Could you check a few things on this model? Use its own coordinates, in mm. A direction names the side the tool comes from. Coordinates: 2 decimals unless noted, no trailing zeros. Write each loop counter-clockwise with the first axis right and the second up, starting at its lowest first coordinate (ties: lowest second). Pieces come first, ordered by that corner, then holes. Notation, with made-up numbers: M 43,-38 L 65,-38 A11 cw 65,-20 Z; hole C -21.75,-36 d4. An arc over 180 degrees is marked long. Write item = value, one per line.
```python
from build123d import *

# Parameters (mm, degrees)
SKETCH4_W               = 40
SKETCH4_H               = 80
BOSS_EXTRUDE4_DEPTH     = 5
SKETCH5_W               = 10
SKETCH5_H               = 5
BOSS_EXTRUDE6_DEPTH     = 50
SKETCH7_W               = 10
SKETCH7_H               = 25
SKETCH7_H_2             = 5
BOSS_EXTRUDE7_DEPTH     = 20
SKETCH8_W               = 40
SKETCH8_H               = 5
BOSS_EXTRUDE8_DEPTH     = 20
SKETCH9_W               = 100
SKETCH9_H               = 5
BOSS_EXTRUDE9_DEPTH     = 10
SKETCH10_W              = 5
SKETCH10_H              = 50
BOSS_EXTRUDE10_DEPTH    = 40
BOSS_EXTRUDE11_DEPTH    = 10
SKETCH12_R              = 15
SKETCH12_R_2            = 1.8
CUT_EXTRUDE1_DEPTH      = 5
CUT_EXTRUDE2_DEPTH      = 92.241437954
CUT_EXTRUDE2_DEPTH_BACK = 92.241437954
SKETCH13_R              = 2.25
SKETCH14_R              = 4
SKETCH14_R_2            = 2.25
CUT_EXTRUDE4_DEPTH      = 2
CUT_EXTRUDE5_START      = -2
SKETCH15_R              = 4
SKETCH15_R_2            = 2.25
CUT_EXTRUDE5_DEPTH      = 2
SKETCH17_R              = 5
CUT_EXTRUDE6_DEPTH      = 25
SKETCH19_W              = 50
SKETCH19_H              = 60
SKETCH19_R              = 1.8
SKETCH19_R_2            = 15
SKETCH19_R_3            = 4
BOSS_EXTRUDE13_DEPTH    = 5
SKETCH20_R              = 4
SKETCH20_R_2            = 2.25
BOSS_EXTRUDE14_DEPTH    = 5
SKETCH21_W              = 20
SKETCH21_H              = 20
BOSS_EXTRUDE15_DEPTH    = 5
BOSS_EXTRUDE16_START    = -10
SKETCH22_R              = 4
BOSS_EXTRUDE16_DEPTH    = 10
SKETCH23_R              = 4
BOSS_EXTRUDE17_DEPTH    = 5
CUT_EXTRUDE7_DEPTH      = 106.59356041
CUT_EXTRUDE7_DEPTH_BACK = 106.59356041
SKETCH24_R              = 2.6
SKETCH25_W              = 55
SKETCH25_H              = 100
BOSS_EXTRUDE18_DEPTH    = 5
SKETCH26_W              = 55
SKETCH26_H              = 10
BOSS_EXTRUDE19_DEPTH    = 20


with BuildPart() as part:
    # Sketch4 → Boss-Extrude4 (new body)
    with BuildSketch(Plane(origin=(0, 0, 0), x_dir=(1, 0, 0), z_dir=(0, 1, 0))):
        with Locations((20, 40)):
            Rectangle(SKETCH4_W, SKETCH4_H)
    extrude(amount=BOSS_EXTRUDE4_DEPTH)

    # Sketch5 → Boss-Extrude6 (add)
    with BuildSketch(Plane(origin=(0, 5, 0), x_dir=(1, 0, 0), z_dir=(0, 1, 0))):
        with Locations((35, 52.5)):
            Rectangle(SKETCH5_W, SKETCH5_H)
        with Locations((35, 27.5)):
            Rectangle(SKETCH5_W, SKETCH5_H)
    extrude(amount=BOSS_EXTRUDE6_DEPTH)

    # Sketch7 → Boss-Extrude7 (add)
    with BuildSketch(Plane.XY.offset(-50)):
        with Locations((35, 17.5)):
            Rectangle(SKETCH7_W, SKETCH7_H)
        with Locations((35, 52.5)):
            Rectangle(SKETCH7_W, SKETCH7_H_2)
    extrude(amount=BOSS_EXTRUDE7_DEPTH)

    # Sketch8 → Boss-Extrude8 (add)
    with BuildSketch(Plane(origin=(0, 0, -80), x_dir=(-1, 0, 0), z_dir=(0, 0, -1))):
        with Locations((-20, 2.5)):
            Rectangle(SKETCH8_W, SKETCH8_H)
    extrude(amount=BOSS_EXTRUDE8_DEPTH)

    # Sketch9 → Boss-Extrude9 (add)
    with BuildSketch(Plane.ZY):
        with Locations((-50, 2.5)):
            Rectangle(SKETCH9_W, SKETCH9_H)
    extrude(amount=BOSS_EXTRUDE9_DEPTH)

    # Sketch10 → Boss-Extrude10 (add)
    with BuildSketch(Plane.ZY.offset(-30)):
        with Locations((-52.5, 30)):
            Rectangle(SKETCH10_W, SKETCH10_H)
    extrude(amount=BOSS_EXTRUDE10_DEPTH)

    # Sketch11 → Boss-Extrude11 (add)
    with BuildSketch(Plane(origin=(0, 55, 0), x_dir=(1, 0, 0), z_dir=(0, 1, 0))):
        Polygon((40, 55), (-10, 55), (-10, 50), (30, 50), (30, 25), (40, 25), align=None)
    extrude(amount=BOSS_EXTRUDE11_DEPTH)

    # Sketch12 → Cut-Extrude1 (cut)
    with BuildSketch(Plane.XY.offset(-50)):
        with Locations((11, 40)):
            Circle(SKETCH12_R)
        with Locations((-4.499780644, 55.499780644)):
            Circle(SKETCH12_R_2)
        with Locations((26.499780644, 55.499780644)):
            Circle(SKETCH12_R_2)
        with Locations((-4.499780644, 24.500219356)):
            Circle(SKETCH12_R_2)
        with Locations((26.499780644, 24.500219356)):
            Circle(SKETCH12_R_2)
    extrude(amount=-CUT_EXTRUDE1_DEPTH, mode=Mode.SUBTRACT)

    # Sketch13 → Cut-Extrude2 (cut, two sides: drawn at the far end of the back side and taken through both)
    with BuildSketch(Plane.XY.offset(-50).offset(-CUT_EXTRUDE2_DEPTH_BACK)):
        with Locations((35, 40)):
            Circle(SKETCH13_R)
    extrude(amount=CUT_EXTRUDE2_DEPTH + CUT_EXTRUDE2_DEPTH_BACK, mode=Mode.SUBTRACT)

    # Sketch14 → Cut-Extrude4 (cut)
    with BuildSketch(Plane.XY.offset(-25)):
        with Locations((35, 40)):
            Circle(SKETCH14_R)
        with Locations((35, 40)):
            Circle(SKETCH14_R_2, mode=Mode.SUBTRACT)
    extrude(amount=-CUT_EXTRUDE4_DEPTH, mode=Mode.SUBTRACT)

    # Sketch15 → Cut-Extrude5 (cut)
    with BuildSketch(Plane(origin=(0, 0, -55), x_dir=(-1, 0, 0), z_dir=(0, 0, -1)).offset(CUT_EXTRUDE5_START)):
        with Locations(Location((-35, 40, 0), (0, 0, 180))):
            Circle(SKETCH15_R)
        with Locations(Location((-35, 40, 0), (0, 0, 180))):
            Circle(SKETCH15_R_2, mode=Mode.SUBTRACT)
    extrude(amount=CUT_EXTRUDE5_DEPTH, mode=Mode.SUBTRACT)

    # Sketch17 → Cut-Extrude6 (cut)
    with BuildSketch(Plane.XY.offset(-25)):
        with Locations((26.499780644, 55.499780644)):
            Circle(SKETCH17_R)
        with Locations((26.499780644, 24.500219356)):
            Circle(SKETCH17_R)
    extrude(amount=-CUT_EXTRUDE6_DEPTH, mode=Mode.SUBTRACT)

    # Sketch19 → Boss-Extrude13 (add)
    with BuildSketch(Plane(origin=(0, 0, -55), x_dir=(-1, 0, 0), z_dir=(0, 0, -1))):
        with Locations((-15, 35)):
            Rectangle(SKETCH19_W, SKETCH19_H)
        with Locations(Location((4.499780644, 55.499780644, 0), (0, 0, 180))):
            Circle(SKETCH19_R, mode=Mode.SUBTRACT)
        with Locations(Location((4.499780644, 24.500219356, 0), (0, 0, 180))):
            Circle(SKETCH19_R, mode=Mode.SUBTRACT)
        with Locations(Location((-26.499780644, 24.500219356, 0), (0, 0, 180))):
            Circle(SKETCH19_R, mode=Mode.SUBTRACT)
        with Locations(Location((-11, 40, 0), (0, 0, 180))):
            Circle(SKETCH19_R_2, mode=Mode.SUBTRACT)
        with Locations(Location((-35, 40, 0), (0, 0, 180))):
            Circle(SKETCH19_R_3, mode=Mode.SUBTRACT)
        with Locations(Location((-26.499780644, 55.499780644, 0), (0, 0, 180))):
            Circle(SKETCH19_R, mode=Mode.SUBTRACT)
    extrude(amount=BOSS_EXTRUDE13_DEPTH)

    # Sketch20 → Boss-Extrude14 (add)
    with BuildSketch(Plane(origin=(0, 0, -53), x_dir=(-1, 0, 0), z_dir=(0, 0, -1))):
        with Locations(Location((-35, 40, 0), (0, 0, 180))):
            Circle(SKETCH20_R)
        with Locations(Location((-35, 40, 0), (0, 0, 180))):
            Circle(SKETCH20_R_2, mode=Mode.SUBTRACT)
    extrude(amount=BOSS_EXTRUDE14_DEPTH)

    # Sketch21 → Boss-Extrude15 (add)
    with BuildSketch(Plane(origin=(40, 0, 0), x_dir=(0, 0, -1), z_dir=(1, 0, 0))):
        Polygon((100, 5), (60, 5), (60, 65), (25, 65), (25, 5), (0, 5), (0, 0), (100, 0), align=None)
        with Locations((40, 40)):
            Rectangle(SKETCH21_W, SKETCH21_H, mode=Mode.SUBTRACT)
    extrude(amount=BOSS_EXTRUDE15_DEPTH)

    # Sketch22 → Boss-Extrude16 (add)
    with BuildSketch(Plane(origin=(0, 0, -60), x_dir=(-1, 0, 0), z_dir=(0, 0, -1)).offset(BOSS_EXTRUDE16_START)):
        with Locations(Location((-35, 40, 0), (0, 0, 180))):
            Circle(SKETCH22_R)
    extrude(amount=BOSS_EXTRUDE16_DEPTH)

    # Sketch23 → Boss-Extrude17 (add)
    with BuildSketch(Plane.XY.offset(-25)):
        with Locations((35, 40)):
            Circle(SKETCH23_R)
    extrude(amount=-BOSS_EXTRUDE17_DEPTH)

    # Sketch24 → Cut-Extrude7 (cut, two sides: drawn at the far end of the back side and taken through both)
    with BuildSketch(Plane(origin=(0, 0, -30), x_dir=(-1, 0, 0), z_dir=(0, 0, -1)).offset(-CUT_EXTRUDE7_DEPTH_BACK)):
        with Locations((-37.5, 40)):
            Circle(SKETCH24_R)
    extrude(amount=CUT_EXTRUDE7_DEPTH + CUT_EXTRUDE7_DEPTH_BACK, mode=Mode.SUBTRACT)

    # Sketch25 → Boss-Extrude18 (add)
    with BuildSketch(Plane.XZ):
        with Locations((17.5, -50)):
            Rectangle(SKETCH25_W, SKETCH25_H)
    extrude(amount=BOSS_EXTRUDE18_DEPTH)

    # Sketch26 → Boss-Extrude19 (add)
    with BuildSketch(Plane.XY):
        with Locations((17.5, 0)):
            Rectangle(SKETCH26_W, SKETCH26_H)
    extrude(amount=BOSS_EXTRUDE19_DEPTH)


solid = part.part
```
Item 1: I'm going to push flat-ended pins straight in: P1, Ø4.5, axis at x = 26.5, y = 24.5, coming from the +Z side; P2, Ø7, axis at y = 43, z = -32, coming from the -X side; P3, Ø12, axis at x = 40.5, y = 41, coming from the -Z side. Where does each tip first touch, or does it pass through?
Numbers:
P1 = -50
P2 = 30
P3 = -60
Item 2: Imagine slicing it at B-B (z = -43.5). Write out the boundary of the cut face in (x, y).
Numbers:
outline = M -10,-5 L 45,-5 L 45,30 L 30,30 L 30,28.07 A5 cw 30,20.93 L 30,5 L -10,5 Z; M 30,50 L 45,50 L 45,65 L 30,65 L 30,59.07 A5 cw 30,51.93 Z
Item 3: For faces 5 (the face through (35.7, 37.6, -30)), 6 (the face through (31.5, 24.4, -37.3)), 7 (the face through (30, 62, -38)), 8 (the face through (37, 35, -25)), 9 (the face through (-10, 4, -40)), which set-ups out of +Z, -Z, +X, -X, +Y, -Y let a thin tool reach every point of the face, with its end or its side?
Numbers:
face_5 = +X, -X
face_6 = +Z, -X
face_7 = +Z, -X, +Y
face_8 = +Z, +X, -X, +Y
face_9 = +Z, -Z, -X, +Y, -Y
Item 4: Imagine slicing it at C-C (x = 11). Write out the boundary of the cut face in (y, z), and give its area (3 significant figures).
Numbers:
outline = M -5,-100 L 5,-100 L 5,-60 L 25,-60 L 25,-50 L 5,-50 L 5,20 L -5,20 Z; M 55,-60 L 65,-60 L 65,-50 L 55,-50 Z
area = 1,500 mm²
Item 5: Imagine slicing it at D-D (y = 13.5). Write out the boundary of the cut face in (x, z).
Numbers:
outline = M -10,-60 L 45,-60 L 45,-25 L 30,-25 L 30,-50 L -10,-50 Z
Item 6: Imagine slicing it at A-A (y = 40). Write out the boundary of the cut face in (x, z).
Numbers:
outline = M -10,-60 L -4,-60 L -4,-50 L -10,-50 Z; M 26,-60 L 34.9,-60 L 34.9,-50 L 26,-50 Z; M 30,-30 L 34.9,-30 L 34.9,-25 L 30,-25 Z; M 40.1,-60 L 45,-60 L 45,-50 L 40.1,-50 Z; M 40.1,-30 L 45,-30 L 45,-25 L 40.1,-25 Z
Item 7: If we mould it in two halves opening along Z, with no side actions, what happens to faces 1 (the face through (37, 50, -40)), 2 (the face through (37, 30, -40)), 3 (the face through (17, 0, -100)), 4 (the face through (31.5, 55.4, -37.3))? For each: pulls with the +Z half, pulls with the -Z half, needs draft (parallel to the pull), parting line crosses it, or undercut.
Numbers:
face_1 = undercut
face_2 = undercut
face_3 = pulls with the -Z half
face_4 = needs draft
Item 8: If I drill on line 1 along X through (y, z) = (40, -56); line 2 along Y through (x, z) = (11, -51); line 3 along Z through (x, y) = (34.5, 49.5), over which ranges is the centre line in solid material (lowest first)?
Numbers:
line_1 = -10 to -4, 26 to 34.9, 40.1 to 45
line_2 = -5 to 25, 55 to 65
line_3 = -60 to -50, -30 to -25
